The listing builds one solid part. Answer for the finished solid, in the listing's coordinates (mm). Round coordinates to 2 decimals unless told otherwise and drop trailing zeros. Write each loop counter-clockwise with the first axis right and the second up, starting at its lowest first coordinate (ties: lowest second). Pieces come first, ordered by that corner, then holes.
(1) A cutting plane is placed at B-B, the plane y = 19. Give the vertices of the cut face in (x, z).
(2) A cutting plane is placed at C-C, the plane z = 5.5. Give the vertices of the cut face in (x, y), and give its area (3 significant figures).
(3) A cutting plane is placed at D-D, the plane y = 59.5. Give the vertices of the cut face in (x, z).
(4) Find the intervals of material crossed by probe 1 along Y at (x, z) = (-12.5, -15.5); probe 2 along X at (y, z) = (9, -11); probe 3 along Y at (x, z) = (-9, 12), in increasing order.
(5) Each of these flat-tipped pins is pushed along its axis until it touches: pin 1 Ø4 at (x, y) = (0.5, 105) entering from -Z; pin 2 Ø12 at (y, z) = (61, -6.5) entering from +X; pin 3 Ø8 at (x, z) = (-4, -18.5) entering from +Y. Where does it stop, or does it pass through?
(6) The mould has two halves that part along Z. Classify faces 1 (the face through (16.046, 17, -12)), 2 (the face through (0, 17, -22.88)), 3 (the face through (-2.07, 63.99, 15.77)): +Z half, -Z half, draft (parallel to the pull), parting line (faces both ways), or undercut.
(7) A cutting plane is placed at A-A, the plane x = 0. Give the vertices of the cut face in (y, z), and give its area (3 significant figures).
from build123d import *

# Parameters (mm, degrees)
F0_R     = 15.904078
F1_DEPTH = 129.794
F2_W     = 31.898258
F2_H     = 22.879753
F3_DEPTH = 34.544
F4_R     = 13.890784
F5_DEPTH = 152.908


with BuildPart() as f1:
    # F0 (on Front) → F1 (new body)
    with BuildSketch(Plane.XZ):
        Circle(F0_R)
    extrude(amount=-F1_DEPTH)

    # F2 (on Front) → F3 (join)
    with BuildSketch(Plane.XZ):
        with Locations((0.097296, -11.439876)):
            Rectangle(F2_W, F2_H)
    extrude(amount=-F3_DEPTH)

    # F4 (on Front) → F5 (join)
    with BuildSketch(Plane.XZ):
        Circle(F4_R)
    extrude(amount=-F5_DEPTH)


solid = f1.part
Solutions:
1. outline: (-15.85, -22.88) - (16.05, -22.88) - (16.05, 0) - (15.9, 0) arc R15.9 ccw (long way) to (-15.85, -1.29) - close
2. outline: (-14.92, 0) - (14.92, 0) - (14.92, 129.79) - (12.76, 129.79) - (12.76, 152.91) - (-12.76, 152.91) - (-12.76, 129.79) - (-14.92, 129.79) - close
2. area: 4,460 mm2
3. outline: circle Ø31.81 at (0, 0)
4. probe 1: y = 0 to 34.54
4. probe 2: x = -15.85 to 16.05
4. probe 3: y = 0 to 129.79
5. pin 1: stops at z = -15.9
5. pin 2: stops at x = 15.9
5. pin 3: stops at y = 129.79
6. face 1: draft
6. face 2: -Z half
6. face 3: parting line
7. outline: (0, -22.88) - (34.54, -22.88) - (34.54, -15.9) - (129.79, -15.9) - (129.79, -13.89) - (152.91, -13.89) - (152.91, 13.89) - (129.79, 13.89) - (129.79, 15.9) - (0, 15.9) - close
7. area: 5,010 mm2
